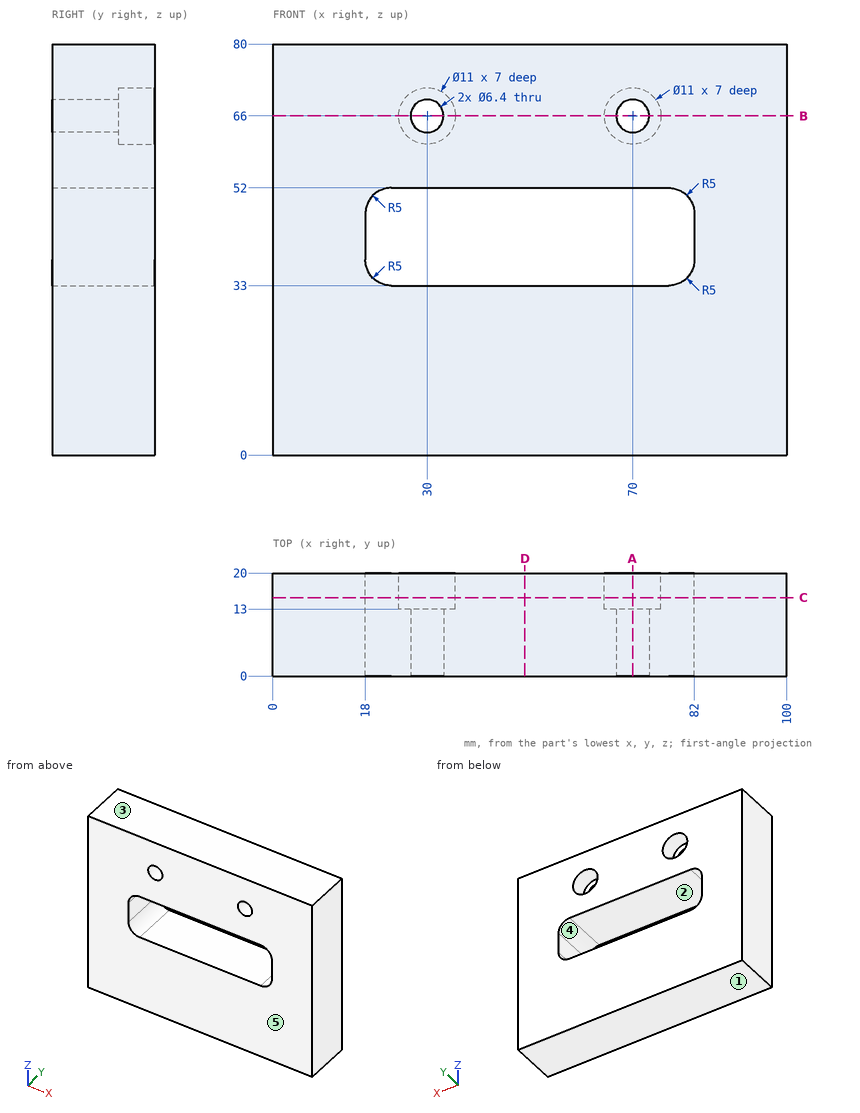
The figure shows three views and two pictorial views of one solid part (mm, origin at its lowest corner). Answer the questions. A direction names the side the tool comes from. Give positions to 0.01 mm unless a question says otherwise; leave off trailing zeros. Order: outer loops, then holes, each group sorted by start corner. A loop starts at its lowest first (then second) coordinate and runs counter-clockwise, first axis right, second up. Notation, with made-up numbers: (-13.5, 1.25) -> (27.5, 1.25) arc R27 ccw to (27.5, 29.25) -> close; hole circle Ø8 at (68.5, 79.5). An arc over 180 degrees is marked (long way). Answer as CSV lines item,"result". Start each with the question number.
(1) Section B-B, the plane z = 66 is taken. Write down the section's boundary in (x, y), plus the area to 3 significant figures.
(2) Consider line 1 along Z through (x, y) = (30, 8); line 2 along X through (y, z) = (4.25, 66); line 3 along Z through (x, y) = (30, 15.75). Determine where each line is inside the solid, lowest interval first.
(3) Section D-D, the plane x = 49 is taken. Write down the section's boundary in (y, z), plus the area to 3 significant figures.
(4) Section C-C, the plane y = 15.25 is taken. Write down the section's boundary in (x, z).
(5) Which of the six approach directions +Z, -Z, +X, -X, +Y, -Y give full straight-line access (tool end or side, diameter ignored) to the marked faces 1 and 2?
(6) For a pull along Z with two mould halves and no side action, classify the marked faces 3, 4 and 5 as released by +Z, released by -Z, zero draft, split by the parting line, or undercut.
(7) Section A-A, the plane x = 70 is taken. Write down the section's boundary in (y, z).
(8) This flat-tipped pin is pushed along its axis until it touches: pin 1 Ø3.5 at (x, z) = (30, 64) entering from +Y. Where does it stop, or does it pass through?
Entries:
1,outline,"(0, 0) -> (26.8, 0) -> (26.8, 13) -> (24.5, 13) -> (24.5, 20) -> (0, 20) -> close; (33.2, 0) -> (66.8, 0) -> (66.8, 13) -> (64.5, 13) -> (64.5, 20) -> (35.5, 20) -> (35.5, 13) -> (33.2, 13) -> close; (73.2, 0) -> (100, 0) -> (100, 20) -> (75.5, 20) -> (75.5, 13) -> (73.2, 13) -> close"
1,area,"1,680 mm²"
2,line 1,"0 to 33, 52 to 62.8, 69.2 to 80"
2,line 2,"0 to 26.8, 33.2 to 66.8, 73.2 to 100"
2,line 3,"0 to 33, 52 to 60.5, 71.5 to 80"
3,outline,"(0, 0) -> (20, 0) -> (20, 33) -> (0, 33) -> close; (0, 52) -> (20, 52) -> (20, 80) -> (0, 80) -> close"
3,area,"1,220 mm²"
4,outline,"(0, 0) -> (100, 0) -> (100, 80) -> (0, 80) -> close; hole (18, 38) arc R5 ccw to (23, 33) -> (77, 33) arc R5 ccw to (82, 38) -> (82, 47) arc R5 ccw to (77, 52) -> (23, 52) arc R5 ccw to (18, 47) -> close; hole circle Ø11 at (30, 66); hole circle Ø11 at (70, 66)"
5,face 1,"-Z, +X, -X, +Y, -Y"
5,face 2,"+Y, -Y"
6,face 3,"released by +Z"
6,face 4,"undercut"
6,face 5,"zero draft"
7,outline,"(0, 0) -> (20, 0) -> (20, 33) -> (0, 33) -> close; (0, 52) -> (20, 52) -> (20, 60.5) -> (13, 60.5) -> (13, 62.8) -> (0, 62.8) -> close; (0, 69.2) -> (13, 69.2) -> (13, 71.5) -> (20, 71.5) -> (20, 80) -> (0, 80) -> close"
8,pin 1,"y = 13"
